Geometry check sheet. Reference: the model listing, model coordinates, mm. Coordinates: 2 decimals unless noted, no trailing zeros. Write each loop counter-clockwise with the first axis right and the second up, starting at its lowest first coordinate (ties: lowest second). Pieces come first, ordered by that corner, then holes. Notation, with made-up numbers: (-2.5, 78) -> (34.5, 78) arc R21 cw to (34.5, 91) -> close; hole circle Ø6 at (31.25, 7). An arc over 180 degrees is marked (long way). Answer in a Markdown table with one row per item. Add a question column.
Q1. Thickness scan on line 1 (X direction, y = -15, z = 2.5); line 2 (X direction, y = -47, z = 1.35); line 3 (Y direction, x = 101.5, z = 0.8). Record the ranges inside material, lowest first.
Q2. Section check C-C, the plane z = 1.25. Record the boundary of the cut face in (x, y) (3 decimals), and give its area (3 significant figures).
Q3. Gauge pin test, flat end, axial feed: P1, Ø3, axis at x = 83.05, y = -47.14, coming from the -Z side. Record the tip position at first contact, or that the pin passes through.
Q4. Section check A-A, the plane y = -27. Record the boundary of the cut face in (x, z).
Q5. Section check B-B, the plane x = 87. Record the boundary of the cut face in (y, z).
```python
from build123d import *

# Parameters (mm, degrees)
CROQUIS1_W              = 72
CROQUIS1_H              = 67
SALIENTE_EXTRUIR1_DEPTH = 3
CROQUIS4_R              = 1.625
CROQUIS4_R_2            = 1.5
CROQUIS4_W              = 26.5
CROQUIS4_H              = 20
CORTAR_EXTRUIR2_DEPTH   = 3


with BuildPart() as part:
    # Croquis1 → Saliente-Extruir1 (new body)
    with BuildSketch(Plane.XY):
        with Locations((83.049688553, -19.639954107)):
            Rectangle(CROQUIS1_W, CROQUIS1_H)
    extrude(amount=SALIENTE_EXTRUIR1_DEPTH)

    # Croquis4 → Cortar-Extruir2 (cut)
    with BuildSketch(Plane(origin=(0, 0, 0), x_dir=(-1, 0, 0), z_dir=(0, 0, -1))):
        with Locations((-83.049688553, -47.139954107)):
            Circle(CROQUIS4_R)
        with Locations((-83.049688553, 10.860045893)):
            Circle(CROQUIS4_R)
        with Locations((-108.049688553, -19.639954107)):
            Circle(CROQUIS4_R_2)
        with Locations((-70.549688553, -19.639954107)):
            Circle(CROQUIS4_R_2)
        with Locations((-89.299688553, -19.639954107)):
            Rectangle(CROQUIS4_W, CROQUIS4_H)
    extrude(amount=-CORTAR_EXTRUIR2_DEPTH, mode=Mode.SUBTRACT)


solid = part.part
```
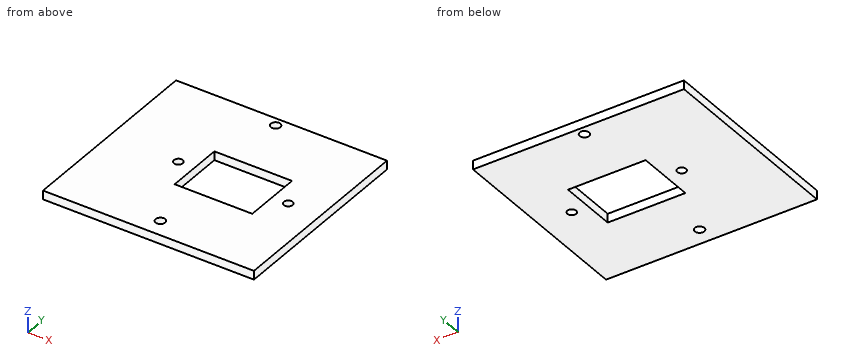
Calculated:
| question | item | result |
|---|---|---|
| 1 | line 1 | x = 47.05 to 76.05, 102.55 to 119.05 |
| 1 | line 2 | x = 47.05 to 81.43, 84.67 to 119.05 |
| 1 | line 3 | y = -53.14 to -29.64, -9.64 to 13.86 |
| 2 | outline | (47.05, -53.14) -> (119.05, -53.14) -> (119.05, 13.86) -> (47.05, 13.86) -> close; hole circle Ø3 at (70.55, -19.64); hole (76.05, -29.64) -> (102.55, -29.64) -> (102.55, -9.64) -> (76.05, -9.64) -> close; hole circle Ø3.25 at (83.05, -47.14); hole circle Ø3.25 at (83.05, 10.86); hole circle Ø3 at (108.05, -19.64) |
| 2 | area | 4,260 mm² |
| 3 | P1 | passes through |
| 4 | outline | (47.05, 0) -> (76.05, 0) -> (76.05, 3) -> (47.05, 3) -> close; (102.55, 0) -> (119.05, 0) -> (119.05, 3) -> (102.55, 3) -> close |
| 5 | outline | (-53.14, 0) -> (-29.64, 0) -> (-29.64, 3) -> (-53.14, 3) -> close; (-9.64, 0) -> (13.86, 0) -> (13.86, 3) -> (-9.64, 3) -> close |
